```python
from build123d import *

# Parameters (mm, degrees)
SKETCH_W        = 60
SKETCH_H        = 60
PAD_DEPTH       = 2
SKETCH001_W     = 55
SKETCH001_H     = 55
PAD001_DEPTH    = 6
SKETCH002_W     = 50
SKETCH002_H     = 50
POCKET_DEPTH    = 2
SKETCH005_W     = 46
SKETCH005_H     = 46
POCKET003_DEPTH = 5
POCKET001_DEPTH = 8.001
SKETCH004_W     = 18
SKETCH004_H     = 5
POCKET002_DEPTH = 7


with BuildPart() as part:
    # Sketch → Pad (new body)
    with BuildSketch(Plane.XY):
        with Locations((30, 30)):
            Rectangle(SKETCH_W, SKETCH_H)
    extrude(amount=PAD_DEPTH)

    # Sketch001 (on DatumPlane) → Pad001 (join)
    with BuildSketch(Plane(origin=(0, 0, 0), x_dir=(1, 0, 0), z_dir=(0, 0, -1))):
        with Locations((30, -30)):
            Rectangle(SKETCH001_W, SKETCH001_H)
    extrude(amount=PAD001_DEPTH)

    # Sketch002 (on DatumPlane) → Pocket (cut)
    with BuildSketch(Plane(origin=(0, 0, -6), x_dir=(1, 0, 0), z_dir=(0, 0, -1))):
        with Locations((30, -30)):
            Rectangle(SKETCH002_W, SKETCH002_H)
    extrude(amount=-POCKET_DEPTH, mode=Mode.SUBTRACT)

    # Sketch005 (on DatumPlane) → Pocket003 (cut)
    with BuildSketch(Plane(origin=(0, 0, -4), x_dir=(1, 0, 0), z_dir=(0, 0, -1))):
        with Locations((30, -30)):
            Rectangle(SKETCH005_W, SKETCH005_H)
    extrude(amount=-POCKET003_DEPTH, mode=Mode.SUBTRACT)

    # Sketch003 (on Face5 of Pocket) → Pocket001 (cut, through all)
    with BuildSketch(Plane.XY.offset(2)):
        Polygon((6.54, 53.46), (34.54, 53.46), (34.54, 45.46), (26.54, 45.46), (26.54, 21.46), (6.54, 21.46), align=None)
    extrude(amount=-POCKET001_DEPTH, mode=Mode.SUBTRACT)

    # Sketch004 (on DatumPlane) → Pocket002 (cut)
    with BuildSketch(Plane(origin=(0, 0, -6), x_dir=(1, 0, 0), z_dir=(0, 0, -1))):
        with Locations((16.54, -5)):
            Rectangle(SKETCH004_W, SKETCH004_H)
    extrude(amount=-POCKET002_DEPTH, mode=Mode.SUBTRACT)


solid = part.part
```
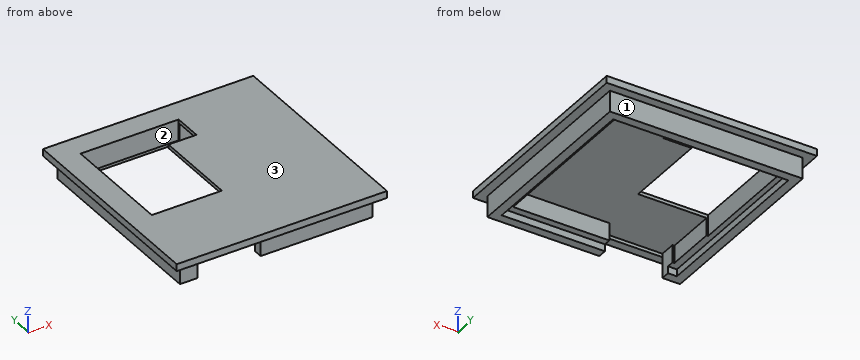
Could you check a few things on this model? Use its own coordinates, in mm. Face numbers are marked on the shaded views. Coordinates: 2 decimals unless noted, no trailing zeros. Write each loop counter-clockwise with the first axis right and the second up, starting at its lowest first coordinate (ties: lowest second). Pieces come first, ordered by that corner, then holes. Notation, with made-up numbers: (69.25, 20.25) - (128.25, 20.25) arc R11 cw to (128.25, 25.25) - close; hole circle Ø2 at (50.25, 74.5). An arc over 180 degrees is marked (long way). Use a Markdown table: item, result.
Q1. Imagine slicing it at C-C (z = -2.75). List the corners of the cut face in (x, y) for me, and give its area (3 significant figures).
Geometry check:
| item | result |
|---|---|
| outline | (2.5, 2.5) - (7.54, 2.5) - (7.54, 7) - (7, 7) - (7, 21.46) - (6.54, 21.46) - (6.54, 53.46) - (34.54, 53.46) - (34.54, 53) - (53, 53) - (53, 7) - (25.54, 7) - (25.54, 2.5) - (57.5, 2.5) - (57.5, 57.5) - (2.5, 57.5) - close |
| area | 801 mm2 |
Q2. I'm going to push flat-ended pins straight in: pin 1 Ø2 at (y, z) = (6, -1.5) entering from +X; pin 2 Ø6 at (x, y) = (33.5, 44) entering from -Z; pin 3 Ø12 at (x, y) = (12, 45) entering from -Z. Where does each tip first touch, or does it pass through?
Geometry check:
| item | result |
|---|---|
| pin 1 | stops at x = 57.5 |
| pin 2 | stops at z = 1 |
| pin 3 | stops at z = -4 |
Q3. Thinking about a two-plate mould opening in Y: for the marked faces 1, 2 and 3, which applies, +Y half, -Y half, draft (parallel to the pull), parting line (faces both ways), or undercut?
Geometry check:
| item | result |
|---|---|
| face 1 | +Y half |
| face 2 | undercut |
| face 3 | draft |
Q4. Imagine slicing it at D-D (y = 4). List the corners of the cut face in (x, z) for me.
Geometry check:
| item | result |
|---|---|
| outline | (0, 0) - (2.5, 0) - (2.5, -6) - (7.54, -6) - (7.54, 1) - (25.54, 1) - (25.54, -6) - (57.5, -6) - (57.5, 0) - (60, 0) - (60, 2) - (0, 2) - close |
Q5. Please list where these lines run through material, in increasing order: L1, parallel to X at y = 22, z = -3.5; L2, parallel to X at y = 39, z = 1.5; L3, parallel to Y at x = 23, z = 1.5.
Geometry check:
| item | result |
|---|---|
| L1 | x = 2.5 to 6.54, 53 to 57.5 |
| L2 | x = 0 to 6.54, 26.54 to 60 |
| L3 | y = 0 to 21.46, 53.46 to 60 |
Q6. Imagine slicing it at A-A (y = 30). List the corners of the cut face in (x, z) for me.
Geometry check:
| item | result |
|---|---|
| outline | (0, 0) - (2.5, 0) - (2.5, -6) - (5, -6) - (5, -4) - (6.54, -4) - (6.54, 2) - (0, 2) - close; (26.54, 1) - (53, 1) - (53, -4) - (55, -4) - (55, -6) - (57.5, -6) - (57.5, 0) - (60, 0) - (60, 2) - (26.54, 2) - close |
Q7. Imagine slicing it at B-B (x = 9). List the corners of the cut face in (y, z) for me, and give its area (3 significant figures).
Geometry check:
| item | result |
|---|---|
| outline | (0, 0) - (2.5, 0) - (2.5, 1) - (21.46, 1) - (21.46, 2) - (0, 2) - close; (53.46, -4) - (55, -4) - (55, -6) - (57.5, -6) - (57.5, 0) - (60, 0) - (60, 2) - (53.46, 2) - close |
| area | 58.2 mm2 |
